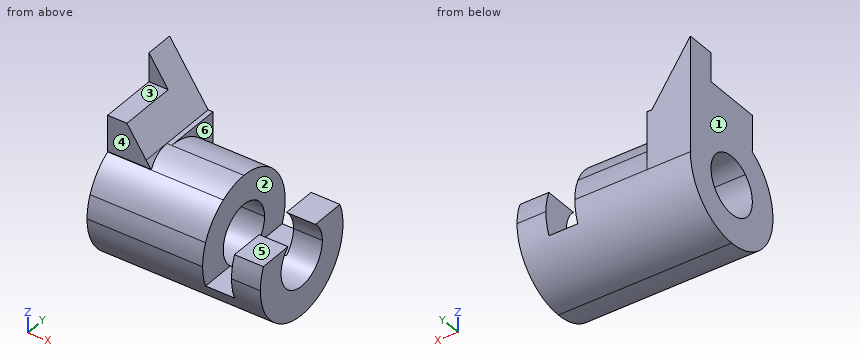
from build123d import *

# Parameters (mm, degrees)
F2_DEPTH  = 25.4
F3_DEPTH  = 254
F4_DEPTH  = 105.41
F5_DEPTH  = 381
F6_DEPTH  = 127
F8_DEPTH  = 19.05
F9_DEPTH  = 12.7
F10_DEPTH = 254


with BuildPart() as f2:
    # F1 (on Front) → F2 (new body, symmetric)
    with BuildSketch(Plane.XZ):
        Polygon((0, -25.4), (0, 0), (0, 9.525), (-12.7, 9.525), (-12.7, -9.525), (-25.4, -9.525), (-25.4, 25.4), (-59.2666666667, 25.4), (-57.15, 22.225), (-76.2, 22.225), (-76.2, -25.4), align=None)
        Polygon((-76.2, 25.4), (-76.2, 22.225), (-57.15, 22.225), (-59.2666666667, 25.4), align=None)
        Polygon((-76.2, 50.8), (-76.2, 25.4), (-59.2666666667, 25.4), align=None)
    extrude(amount=F2_DEPTH, both=True)

    # F0 (on Right) → F3 (cut)
    with BuildSketch(Plane.YZ):
        with BuildLine():
            ThreePointArc((-8.4002604126, 9.525), (-5.2252604126, -11.5752604126), (12.7, 0))
            ThreePointArc((12.7, 0), (11.5752604126, 5.2252604126), (8.4002604126, 9.525))
            ThreePointArc((8.4002604126, 9.525), (0, 12.7), (-8.4002604126, 9.525))
        make_face()
    extrude(amount=-F3_DEPTH, mode=Mode.SUBTRACT)

    # F0 (on Right) → F4 (cut)
    with BuildSketch(Plane.YZ):
        with BuildLine():
            ThreePointArc((-12.7, 21.9970452561), (-6.5740037456, 24.5345159877), (0, 25.4))
            Line((0, 25.4), (-12.7, 25.4))
            Line((-12.7, 25.4), (-12.7, 21.9970452561))
        make_face()
        with BuildLine():
            ThreePointArc((-25.4, 0), (-24.9323016085, 4.8518384664), (-23.5464301965, 9.525))
            ThreePointArc((-23.5464301965, 9.525), (-19.1660873346, 16.6679661712), (-12.7, 21.9970452561))
            Line((-12.7, 21.9970452561), (-12.7, 25.4))
            Line((-12.7, 25.4), (-25.4, 25.4))
            Line((-25.4, 25.4), (-25.4, 0))
        make_face()
    extrude(amount=-F4_DEPTH, mode=Mode.SUBTRACT)

    # F0 (on Right) → F5 (cut)
    with BuildSketch(Plane.YZ):
        with BuildLine():
            ThreePointArc((0, 25.4), (14.1990316571, 21.0605674188), (23.5464301965, 9.525))
            ThreePointArc((23.5464301965, 9.525), (24.9323016085, 4.8518384664), (25.4, 0))
            Line((25.4, 0), (25.4, 25.4))
            Line((25.4, 25.4), (0, 25.4))
        make_face()
    extrude(amount=-F5_DEPTH, mode=Mode.SUBTRACT)

    # F0 (on Right) → F6 (cut)
    with BuildSketch(Plane.YZ):
        Polygon((-25.4, 25.4), (-12.7, 25.4), (-12.7, 38.1), (12.7, 38.1), (12.7, 50.8), (-25.4, 50.8), align=None)
    extrude(amount=-F6_DEPTH, mode=Mode.SUBTRACT)

    # F7 (on face) → F8 (join)
    with BuildSketch(Plane(origin=(-76.2, 0, 0), x_dir=(0, -1, 0), z_dir=(-1, 0, 0))):
        with BuildLine():
            Line((0, 25.4), (-25.4, 25.4))
            Line((-25.4, 25.4), (-25.4, 0))
            ThreePointArc((-25.4, 0), (-17.9605122421, 17.9605122421), (0, 25.4))
        make_face()
    extrude(amount=-F8_DEPTH)

    # F1 (on Front) → F9 (join)
    with BuildSketch(Plane.XZ):
        Polygon((-76.2, 25.4), (-76.2, 22.225), (-57.15, 22.225), (-59.2666666667, 25.4), align=None)
    extrude(amount=F9_DEPTH)

    # F0 (on Right) → F10 (cut)
    with BuildSketch(Plane.YZ):
        with BuildLine():
            ThreePointArc((0, -25.4), (-17.9605122421, -17.9605122421), (-25.4, 0))
            Line((-25.4, 0), (-25.4, -25.4))
            Line((-25.4, -25.4), (0, -25.4))
        make_face()
        with BuildLine():
            Line((25.4, -25.4), (25.4, 0))
            ThreePointArc((25.4, 0), (17.9605122421, -17.9605122421), (0, -25.4))
            Line((0, -25.4), (25.4, -25.4))
        make_face()
    extrude(amount=-F10_DEPTH, mode=Mode.SUBTRACT)


solid = f2.part
Here's how the part is built. I have some questions about the finished solid (model axes, mm). Face numbers are marked on the shaded views. A direction names the side the tool comes from. Coordinates: 2 decimals unless noted, no trailing zeros. Write each loop counter-clockwise with the first axis right and the second up, starting at its lowest first coordinate (ties: lowest second). Pieces come first, ordered by that corner, then holes.
Item 1: I want a section at A-A on x = -63. Write out the boundary of the cut face in (y, z) (3 decimals), and give its area (3 significant figures).
Item 2: If we mould it in two halves opening along X, with no side actions, what happens to the marked faces 1, 2 and 3? For each: +X half, -X half, draft (parallel to the pull), parting line (faces both ways), or undercut.
Item 3: If I drill on line 1 (Z direction, x = -58.5, y = 0); line 2 (X direction, y = 22, z = -6), over which ranges is the centre line in solid material (lowest first)?
Item 4: I want a section at D-D on z = -11. Write out the boundary of the cut face in (x, y).
Item 5: I want a section at C-C on y = 2. Write out the boundary of the cut face in (x, z), and give its area (3 significant figures).
Item 6: On a 3-axis mill with a long thin cutter (end or side, diameter ignored), from which of +Z, -Z, +X, -X, +Y, -Y can I reach the whole of each face in a straight line? I mean the marked faces 4, 5 and 6. Say none if no direction works.
Item 7: Will these pins go through, and if not, where does the flat tip stop? pin 1 (12.5 mm diameter, centred on x = -63.5, z = 27, fed in from -Y); pin 2 (8 mm diameter, centred on x = -44.5, y = 9.5, fed in from -Z); pin 3 (10 mm diameter, centred on x = -12.5, z = 8.5, fed in from -Y).
Item 8: I want a section at B-B on y = 11. Write out the boundary of the cut face in (x, z) (3 decimals).
Findings below:
1. outline: (-12.7, 22.225) - (-12.297, 22.225) arc R25.4 ccw (long way) to (25.4, 0) - (25.4, 31) - (-12.7, 31) - close; hole circle Ø25.4 at (0, 0)
1. area: 1,890 mm2
2. face 1: -X half
2. face 2: undercut
2. face 3: draft
3. line 1: z = -25.4 to -12.7, 12.7 to 25.4
3. line 2: x = -76.2 to -25.4, -12.7 to 0
4. outline: (-76.2, -22.89) - (0, -22.89) - (0, -6.35) - (-76.2, -6.35) - close; (-76.2, 6.35) - (0, 6.35) - (0, 22.89) - (-76.2, 22.89) - close
5. outline: (-76.2, -25.32) - (0, -25.32) - (0, -12.54) - (-76.2, -12.54) - close; (-76.2, 12.54) - (-25.4, 12.54) - (-25.4, 25.32) - (-57.15, 25.32) - (-57.15, 25.4) - (-59.27, 25.4) - (-67.73, 38.1) - (-76.2, 38.1) - close
5. area: 1,790 mm2
6. face 4: +Z, +X, -X, -Y
6. face 5: +Z, +X, +Y, -Y
6. face 6: +Z, +X, +Y
7. pin 1: stops at y = -14.65
7. pin 2: stops at z = -24.8
7. pin 3: stops at y = -25.16
8. outline: (-76.2, -22.895) - (0, -22.895) - (0, -6.347) - (-12.7, -6.347) - (-12.7, -9.525) - (-25.4, -9.525) - (-25.4, -6.347) - (-76.2, -6.347) - close; (-76.2, 6.347) - (-25.4, 6.347) - (-25.4, 22.895) - (-57.15, 22.895) - (-57.15, 25.4) - (-59.267, 25.4) - (-67.733, 38.1) - (-76.2, 38.1) - close; (-12.7, 6.347) - (0, 6.347) - (0, 9.525) - (-12.7, 9.525) - close
